```python
from build123d import *

# Parameters (mm, degrees)
SKETCH1_W           = 50.926738498
SKETCH1_H           = 6.35
SKETCH1_W_2         = 50.926738497
BOSS_EXTRUDE1_DEPTH = 6.35


with BuildPart() as part:
    # Sketch1 → Boss-Extrude1 (new body)
    with BuildSketch(Plane.XY):
        Polygon((-2.593337475, -25.401893638), (-2.593337475, 76.198106362), (-78.793337475, 76.198106362), (-78.793337475, -25.401893638), (-68.658315464, -25.401893638), (-17.731576967, -25.401893638), align=None)
        Polygon((73.606662525, 76.198106362), (-2.593337475, 76.198106362), (-2.593337475, -25.401893638), (12.544902016, -25.401893638), (63.471640514, -25.401893638), (73.606662525, -25.401893638), align=None)
        with Locations((38.008271265, -28.576893638)):
            Rectangle(SKETCH1_W, SKETCH1_H)
        with Locations((-43.194946215, -28.576893638)):
            Rectangle(SKETCH1_W_2, SKETCH1_H)
    extrude(amount=BOSS_EXTRUDE1_DEPTH)


solid = part.part
```
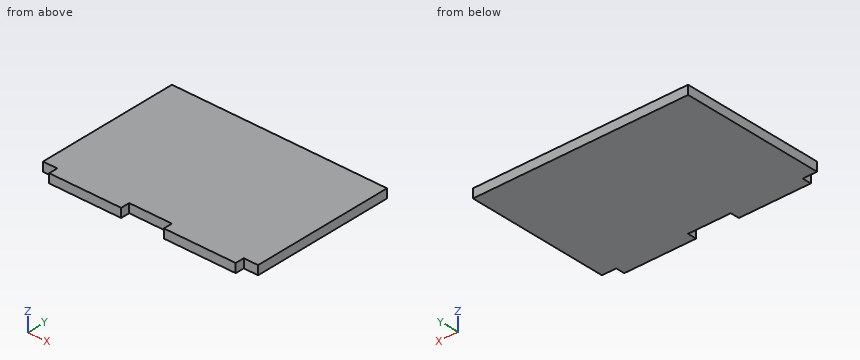
The model under review builds one solid part; all positions refer to its coordinate system, in mm. Round coordinates to 2 decimals unless told otherwise and drop trailing zeros. Loops run counter-clockwise (first coordinate to the right, second up) from the corner with the lowest first, then second, coordinate; pieces in that order, holes last. Notation, with made-up numbers: (83, 4.25) -> (92, 4.25) arc R9 cw to (92, 9.25) -> close; hole circle Ø8 at (-20, 44). An arc over 180 degrees is marked (long way). Answer as a JSON object with one key per item and string values. Group by question number.
1) For pin 1 Ø3 at (x, z) = (-7.5, 3.5) entering from -Y; pin 2 Ø3 at (y, z) = (-29.5, 4) entering from -X, all flat-tipped, find the tip position at first contact; note any pin that passes through.
2) For line 1 (Y direction, x = -69, z = 1.75), list the stretches that pass through material, from the lowest coordinate up. Write a range as [from, to].
3) We need section A-A on z = 3.75. Write out the cut boundary in (x, y), then the cut area to 3 significant figures.
4) We need section B-B on x = 1. Write out the cut boundary in (y, z), then the cut area to 3 significant figures.
Result set:
{
 "1": {"pin 1": "y = -25.4", "pin 2": "x = -68.66"},
 "2": {"line 1": "[-25.4, 76.2]"},
 "3": {"outline": "(-78.79, -25.4) -> (-68.66, -25.4) -> (-68.66, -31.75) -> (-17.73, -31.75) -> (-17.73, -25.4) -> (12.54, -25.4) -> (12.54, -31.75) -> (63.47, -31.75) -> (63.47, -25.4) -> (73.61, -25.4) -> (73.61, 76.2) -> (-78.79, 76.2) -> close", "area": "16,100 mm²"},
 "4": {"outline": "(-25.4, 0) -> (76.2, 0) -> (76.2, 6.35) -> (-25.4, 6.35) -> close", "area": "645 mm²"}
}
